Source: CAD feature listing. Evaluate the final solid. Frame: model axes, mm. A direction names the side the tool comes from. Give positions to 0.01 mm unless a question says otherwise; leave off trailing zeros. Loops run counter-clockwise (first coordinate to the right, second up) from the corner with the lowest first, then second, coordinate; pieces in that order, holes last.
```python
from build123d import *

# Parameters (mm, degrees)
SKETCH1_W           = 58
SKETCH1_H           = 150
BOSS_EXTRUDE1_DEPTH = 3
SKETCH2_R           = 8.076191979
SKETCH2_R_2         = 7.076191979
EXTRUDE_THIN1_DEPTH = 2


with BuildPart() as part:
    # Sketch1 → Boss-Extrude1 (new body)
    with BuildSketch(Plane.XY):
        with Locations((81.977207271, 14.773129951)):
            Rectangle(SKETCH1_W, SKETCH1_H)
    extrude(amount=BOSS_EXTRUDE1_DEPTH)

    # Sketch2 → Extrude-Thin1 (add)
    with BuildSketch(Plane(origin=(0, 79.773129951, 0), x_dir=(1, 0, 0), z_dir=(0, 1, 0))):
        with Locations((81.977207271, -9.724450767)):
            Circle(SKETCH2_R)
        with Locations((81.977207271, -9.724450767)):
            Circle(SKETCH2_R_2, mode=Mode.SUBTRACT)
    extrude(amount=EXTRUDE_THIN1_DEPTH)


solid = part.part
```
(1) Section C-C, the plane y = 9.5. Return the cut outline in (x, z), then the cut area to 3 significant figures.
A:
outline: (52.98, 0) - (110.98, 0) - (110.98, 3) - (52.98, 3) - close
area: 174 mm2
(2) Section B-B, the plane x = 81.5. Return the cut outline in (y, z).
A:
outline: (-60.23, 0) - (89.77, 0) - (89.77, 3) - (-60.23, 3) - close; (79.77, 16.78) - (81.77, 16.78) - (81.77, 17.79) - (79.77, 17.79) - close
(3) Section A-A, the plane z = 6.25. Return the cut outline in (x, y), then the cut area to 3 significant figures.
A:
outline: (74.69, 79.77) - (75.81, 79.77) - (75.81, 81.77) - (74.69, 81.77) - close; (88.14, 79.77) - (89.27, 79.77) - (89.27, 81.77) - (88.14, 81.77) - close
area: 4.50 mm2
(4) Reachability of faces 1 (the flat face through (86, 81.773, 16)), 2 (the flat face through (52.977, 14, 1)) from +Z, -Z, +X, -X, +Y, -Y: full face, straight path, thin tool, end or side. Return the list, or none.
A:
face 1: +Z, +X, -X, +Y
face 2: +Z, -Z, -X, +Y, -Y
(5) Mould query, pull axis Z, two halves, no side actions, for faces 3 (the flat face through (82, 16, 0)), 4 (the flat face through (86, 79.773, 16)), 5 (the cylindrical face through (81.688, 80.759, 17.795)). Classes: pulls with the +Z half, pulls with the -Z half, needs draft (parallel to the pull), parting line crosses it, or undercut.
A:
face 3: pulls with the -Z half
face 4: needs draft
face 5: undercut
(6) Ray query, line 1 along Y through (x, z) = (75, 12.5); line 2 along Z through (x, y) = (83, -17). Return the intervals inside material, ascending.
A:
line 1: y = 79.77 to 81.77
line 2: z = 0 to 3
(7) Section D-D, the plane x = 57.5. Return the cut outline in (y, z).
A:
outline: (-60.23, 0) - (89.77, 0) - (89.77, 3) - (-60.23, 3) - close
(8) First-contact query: pin 1 (8 mm diameter, centred on x = 75, z = 8, fed in from -Y); pin 2 (4 mm diameter, centred on x = 87.5, y = -10.5, fed in from +Z). Flat tips, straight axial feed; report the tip coordinate or a pass-through.
A:
pin 1: stops at y = 79.77
pin 2: stops at z = 3
